from build123d import *

# Parameters (mm, degrees)
F0_W     = 355.6
F0_H     = 254
F1_DEPTH = 6.35
F2_SIZE2 = 6.34999
F2_SIZE  = 6.34999


# Not quite as in the source:
# - a fillet or chamfer is up to 0.001 mm smaller than in the source, because OpenCascade refuses the exact size


with BuildPart() as f1:
    # F0 (on Front) → F1 (new body)
    with BuildSketch(Plane.XZ):
        with Locations((-3.309763968, 6.3614202906)):
            Rectangle(F0_W, F0_H)
    extrude(amount=F1_DEPTH)

    # F2 (size 6.35 and 6.35 in the source; OpenCascade refuses exactly that, so slightly less here)
    f2_edges = [f1.edges().sort_by_distance(p)[0] for p in [
        (-3.309764, -6.35, 133.36142),
        (-181.109764, -6.35, 6.36142),
        (-3.309764, -6.35, -120.63858),
        (174.490236, -6.35, 6.36142),
    ]]
    chamfer(f2_edges, length=F2_SIZE, length2=F2_SIZE2)


solid = f1.part
Here's how the part is built. I have some questions about the finished solid (model axes, mm). Round coordinates to 2 decimals unless told otherwise and drop trailing zeros. Order: outer loops, then holes, each group sorted by start corner. A loop starts at its lowest first (then second) coordinate and runs counter-clockwise, first axis right, second up. Notation, with made-up numbers: (36.5, -20) -> (45.5, -20) arc R22 cw to (45.5, -1) -> close; hole circle Ø11 at (28, 22). An arc over 180 degrees is marked (long way). Use CSV: the item, a comma, the result in double quotes.
1. I need wall thicknesses on line 1 along Z through (x, y) = (37.5, -1.5); line 2 along Z through (x, y) = (153, -2.75); line 3 along X through (y, z) = (-4.5, 83.5). Which ranges of each line are inside material? Lowest first, please.
Recorded:
line 1,"z = -119.14 to 131.86"
line 2,"z = -117.89 to 130.61"
line 3,"x = -176.61 to 169.99"
2. I'm going to push flat-ended pins straight in: P1, Ø2, axis at x = 40, y = -5, coming from the +Z side; P2, Ø1, axis at x = -98, y = -1.5, coming from the -Z side; P3, Ø2, axis at x = -125.5, y = -3.5, coming from the -Z side. Where does each tip first touch, or does it pass through?
Recorded:
P1,"stops at z = 129.36"
P2,"stops at z = -119.64"
P3,"stops at z = -118.14"
3. I want a section at C-C on y = -5. List the corners of the cut face in (x, z) for me.
Recorded:
outline,"(-176.11, -115.64) -> (169.49, -115.64) -> (169.49, 128.36) -> (-176.11, 128.36) -> close"
